```python
from build123d import *

# Parameters (mm, degrees)
BOSS_EXTRUDE1_DEPTH = 5
CUT_EXTRUDE1_DEPTH  = 5
CUT_EXTRUDE2_DEPTH  = 5
SKETCH7_R           = 1.5
CUT_EXTRUDE3_DEPTH  = 5
CUT_EXTRUDE4_DEPTH  = 5
SKETCH10_R          = 1.5
CUT_EXTRUDE5_DEPTH  = 5
CUT_EXTRUDE6_DEPTH  = 5
CUT_EXTRUDE7_DEPTH  = 5


with BuildPart() as part:
    # Sketch1 → Boss-Extrude1 (new body)
    with BuildSketch(Plane(origin=(0, 0, 0), x_dir=(1, 0, 0), z_dir=(0, 1, 0))):
        with BuildLine():
            Line((-4.859778007, 4.413916891), (128.140221993, 4.413916891))
            ThreePointArc((128.140221993, 4.413916891), (128.847328775, 4.121023672), (129.140221993, 3.413916891))
            Line((129.140221993, 3.413916891), (129.140221993, -144.586083109))
            ThreePointArc((129.140221993, -144.586083109), (128.847328775, -145.29318989), (128.140221993, -145.586083109))
            Line((128.140221993, -145.586083109), (-4.859778007, -145.586083109))
            ThreePointArc((-4.859778007, -145.586083109), (-5.566884788, -145.29318989), (-5.859778007, -144.586083109))
            Line((-5.859778007, -144.586083109), (-5.859778007, 3.413916891))
            ThreePointArc((-5.859778007, 3.413916891), (-5.566884788, 4.121023672), (-4.859778007, 4.413916891))
        make_face()
    extrude(amount=BOSS_EXTRUDE1_DEPTH)

    # Sketch3 → Cut-Extrude1 (cut)
    with BuildSketch(Plane(origin=(75.20450804, 5, 34.196611672), x_dir=(1, 0, 0), z_dir=(0, 1, 0))):
        with BuildLine():
            Line((45.935713953, -83.389471436), (45.935713953, -41.389471436))
            ThreePointArc((45.935713953, -41.389471436), (47.435713953, -39.889471436), (48.935713953, -41.389471436))
            Line((48.935713953, -41.389471436), (48.935713953, -83.389471436))
            ThreePointArc((48.935713953, -83.389471436), (47.435713953, -84.889471436), (45.935713953, -83.389471436))
        make_face()
        with BuildLine():
            Line((45.935713953, -31.389471436), (45.935713953, 10.610528564))
            ThreePointArc((45.935713953, 10.610528564), (47.435713953, 12.110528564), (48.935713953, 10.610528564))
            Line((48.935713953, 10.610528564), (48.935713953, -31.389471436))
            ThreePointArc((48.935713953, -31.389471436), (47.435713953, -32.889471436), (45.935713953, -31.389471436))
        make_face()
        with BuildLine():
            Line((-73.064286047, -84.889471436), (-73.064286047, -42.889471436))
            ThreePointArc((-73.064286047, -42.889471436), (-74.564286047, -41.389471436), (-76.064286047, -42.889471436))
            Line((-76.064286047, -42.889471436), (-76.064286047, -84.889471436))
            ThreePointArc((-76.064286047, -84.889471436), (-74.564286047, -86.389471436), (-73.064286047, -84.889471436))
        make_face()
        with BuildLine():
            Line((-73.064286047, -32.889471436), (-73.064286047, 9.110528564))
            ThreePointArc((-73.064286047, 9.110528564), (-74.564286047, 10.610528564), (-76.064286047, 9.110528564))
            Line((-76.064286047, 9.110528564), (-76.064286047, -32.889471436))
            ThreePointArc((-76.064286047, -32.889471436), (-74.564286047, -34.389471436), (-73.064286047, -32.889471436))
        make_face()
    extrude(amount=-CUT_EXTRUDE1_DEPTH, mode=Mode.SUBTRACT)

    # Sketch5 → Cut-Extrude2 (cut)
    with BuildSketch(Plane(origin=(75.20450804, 5, 34.196611672), x_dir=(1, 0, 0), z_dir=(0, 1, 0))):
        with BuildLine():
            Line((-60.064286047, -99.389471436), (-18.064286047, -99.389471436))
            ThreePointArc((-18.064286047, -99.389471436), (-16.564286047, -100.889471436), (-18.064286047, -102.389471436))
            Line((-18.064286047, -102.389471436), (-60.064286047, -102.389471436))
            ThreePointArc((-60.064286047, -102.389471436), (-61.564286047, -100.889471436), (-60.064286047, -99.389471436))
        make_face()
        with BuildLine():
            Line((-9.064286047, -99.389471436), (32.935713953, -99.389471436))
            ThreePointArc((32.935713953, -99.389471436), (34.435713953, -100.889471436), (32.935713953, -102.389471436))
            Line((32.935713953, -102.389471436), (-9.064286047, -102.389471436))
            ThreePointArc((-9.064286047, -102.389471436), (-10.564286047, -100.889471436), (-9.064286047, -99.389471436))
        make_face()
    extrude(amount=-CUT_EXTRUDE2_DEPTH, mode=Mode.SUBTRACT)

    # Sketch7 → Cut-Extrude3 (cut)
    with BuildSketch(Plane(origin=(75.20450804, 5, 34.196611672), x_dir=(1, 0, 0), z_dir=(0, 1, 0))):
        with Locations(Location((44.935713953, -98.389471436, 0), (0, 0, 270))):
            Circle(SKETCH7_R)
        with Locations(Location((44.935713953, 25.610528564, 0), (0, 0, 90))):
            Circle(SKETCH7_R)
        with Locations(Location((-74.064286047, 25.610528564, 0), (0, 0, 270))):
            Circle(SKETCH7_R)
        with BuildLine():
            Line((-72.564286047, -96.712473991), (-72.564286047, -100.066468882))
            ThreePointArc((-72.564286047, -100.066468882), (-74.064286047, -101.566468882), (-75.564286047, -100.066468882))
            Line((-75.564286047, -100.066468882), (-75.564286047, -96.712473991))
            ThreePointArc((-75.564286047, -96.712473991), (-74.064286047, -95.212473991), (-72.564286047, -96.712473991))
        make_face()
    extrude(amount=-CUT_EXTRUDE3_DEPTH, mode=Mode.SUBTRACT)

    # Sketch9 → Cut-Extrude4 (cut)
    with BuildSketch(Plane(origin=(75.20450804, 5, 34.196611672), x_dir=(1, 0, 0), z_dir=(0, 1, 0))):
        with BuildLine():
            Line((-40.064286047, -36.389471436), (12.935713953, -36.389471436))
            ThreePointArc((12.935713953, -36.389471436), (13.642820734, -36.682364655), (13.935713953, -37.389471436))
            Line((13.935713953, -37.389471436), (13.935713953, -55.389471436))
            ThreePointArc((13.935713953, -55.389471436), (13.642820734, -56.096578218), (12.935713953, -56.389471436))
            Line((12.935713953, -56.389471436), (-40.064286047, -56.389471436))
            ThreePointArc((-40.064286047, -56.389471436), (-40.771392828, -56.096578218), (-41.064286047, -55.389471436))
            Line((-41.064286047, -55.389471436), (-41.064286047, -37.389471436))
            ThreePointArc((-41.064286047, -37.389471436), (-40.771392828, -36.682364655), (-40.064286047, -36.389471436))
        make_face()
    extrude(amount=-CUT_EXTRUDE4_DEPTH, mode=Mode.SUBTRACT)

    # Sketch10 → Cut-Extrude5 (cut)
    with BuildSketch(Plane(origin=(0, 5, 0), x_dir=(1, 0, 0), z_dir=(0, 1, 0))):
        with Locations(Location((36.640221993, -5.586083109, 0), (0, 0, 270))):
            Circle(SKETCH10_R)
        with Locations(Location((86.640221993, -5.586083109, 0), (0, 0, 270))):
            Circle(SKETCH10_R)
        with Locations(Location((86.640221993, -55.586083109, 0), (0, 0, 270))):
            Circle(SKETCH10_R)
        with Locations(Location((36.640221993, -55.586083109, 0), (0, 0, 270))):
            Circle(SKETCH10_R)
    extrude(amount=-CUT_EXTRUDE5_DEPTH, mode=Mode.SUBTRACT)

    # Sketch11 → Cut-Extrude6 (cut)
    with BuildSketch(Plane(origin=(0, 5, 0), x_dir=(1, 0, 0), z_dir=(0, 1, 0))):
        with BuildLine():
            Line((32.140221993, -25.086083109), (32.140221993, -119.086083109))
            ThreePointArc((32.140221993, -119.086083109), (30.640221993, -120.586083109), (29.140221993, -119.086083109))
            Line((29.140221993, -119.086083109), (29.140221993, -25.086083109))
            ThreePointArc((29.140221993, -25.086083109), (30.640221993, -23.586083109), (32.140221993, -25.086083109))
        make_face()
        with BuildLine():
            Line((91.140221993, -25.086083109), (91.140221993, -119.086083109))
            ThreePointArc((91.140221993, -119.086083109), (92.640221993, -120.586083109), (94.140221993, -119.086083109))
            Line((94.140221993, -119.086083109), (94.140221993, -25.086083109))
            ThreePointArc((94.140221993, -25.086083109), (92.640221993, -23.586083109), (91.140221993, -25.086083109))
        make_face()
    extrude(amount=-CUT_EXTRUDE6_DEPTH, mode=Mode.SUBTRACT)

    # Sketch12 → Cut-Extrude7 (cut)
    with BuildSketch(Plane(origin=(0, 5, 0), x_dir=(1, 0, 0), z_dir=(0, 1, 0))):
        with BuildLine():
            Line((22.394580423, -97.440920872), (8.394580423, -97.440920872))
            ThreePointArc((8.394580423, -97.440920872), (7.687473642, -97.148027653), (7.394580423, -96.440920872))
            Line((7.394580423, -96.440920872), (7.394580423, -88.440920872))
            ThreePointArc((7.394580423, -88.440920872), (7.687473642, -87.733814091), (8.394580423, -87.440920872))
            Line((8.394580423, -87.440920872), (22.394580423, -87.440920872))
            ThreePointArc((22.394580423, -87.440920872), (23.101687204, -87.733814091), (23.394580423, -88.440920872))
            Line((23.394580423, -88.440920872), (23.394580423, -96.440920872))
            ThreePointArc((23.394580423, -96.440920872), (23.101687204, -97.148027653), (22.394580423, -97.440920872))
        make_face()
        with BuildLine():
            Line((100.885863564, -87.440920872), (114.885863564, -87.440920872))
            ThreePointArc((114.885863564, -87.440920872), (115.592970345, -87.733814091), (115.885863564, -88.440920872))
            Line((115.885863564, -88.440920872), (115.885863564, -96.440920872))
            ThreePointArc((115.885863564, -96.440920872), (115.592970345, -97.148027653), (114.885863564, -97.440920872))
            Line((114.885863564, -97.440920872), (100.885863564, -97.440920872))
            ThreePointArc((100.885863564, -97.440920872), (100.178756783, -97.148027653), (99.885863564, -96.440920872))
            Line((99.885863564, -96.440920872), (99.885863564, -88.440920872))
            ThreePointArc((99.885863564, -88.440920872), (100.178756783, -87.733814091), (100.885863564, -87.440920872))
        make_face()
    extrude(amount=-CUT_EXTRUDE7_DEPTH, mode=Mode.SUBTRACT)


solid = part.part
```
The listing builds one solid part. Answer for the finished solid, in the listing's coordinates (mm). A direction names the side the tool comes from. Give positions to 0.01 mm unless a question says otherwise; leave off trailing zeros. Loops run counter-clockwise (first coordinate to the right, second up) from the corner with the lowest first, then second, coordinate; pieces in that order, holes last. Notation, with made-up numbers: (61.5, 17) - (101.5, 17) arc R23 ccw to (101.5, 45) - close; hole circle Ø4 at (-23.75, -27.5). An arc over 180 degrees is marked (long way). Return JSON: item names as keys, results as strings. Group by question number.
1. Find section B-B (x = 69). Write down the section's boundary in (y, z), then the cut area to 3 significant figures.
2. Straight lines are drawn through the part: line 1 (X direction, y = 4.7, z = 63.5); line 2 (Z direction, x = 108, y = 1.9); line 3 (X direction, y = 2.2, z = 81). For each, find the intervals that lie inside material, in ascending order. Write a range as [from, to].
3. Find section D-D (y = 2.6). State how many separate pieces and enclosed holes the cut face has, then the cut area to 3 significant figures.
4. Determine the mould class of faces 3 (the flat face through (62, 3, 90.586)), 4 (the flat face through (124.14, 3, 44)), 5 (the flat face through (63, 2, 145.586)) for opening direction X: pulls with the +X half, pulls with the -X half, needs draft (parallel to the pull), parting line crosses it, or undercut.
5. Find section C-C (x = 105.5). Write down the section's boundary in (y, z), then the cut area to 3 significant figures.
6. Given pin 1 Ø2 at (x, z) = (42, 13.5) entering from -Y, flat-ended and moving along its own axis, determine where the tip first touches the part or whether it passes through.
7. Find section A-A (z = 29). Write down the section's boundary in (x, y), then the cut area to 3 significant figures.
8. Which of the six approach directions +Z, -Z, +X, -X, +Y, -Y give full straight-line access (tool end or side, diameter ignored) to faces 1 (the flat face through (124.14, 3, 96)), 2 (the flat face through (63, 0, 70))?
Verdict:
{
 "1": {"outline": "(0, -4.41) - (5, -4.41) - (5, 70.59) - (0, 70.59) - close; (0, 90.59) - (5, 90.59) - (5, 133.59) - (0, 133.59) - close; (0, 136.59) - (5, 136.59) - (5, 145.59) - (0, 145.59) - close", "area": "635 mm^2"},
 "2": {"line 1": "x = [-5.86, -0.86], [2.14, 29.14], [32.14, 91.14], [94.14, 121.14], [124.14, 129.14]", "line 2": "z = [-4.41, 87.44], [97.44, 133.59], [136.59, 145.59]", "line 3": "x = [-5.86, -0.86], [2.14, 29.14], [32.14, 34.14], [89.14, 91.14], [94.14, 121.14], [124.14, 129.14]"},
 "3": {"separate pieces": "1", "enclosed holes": "19", "area": "17,400 mm^2"},
 "4": {"face 3": "undercut", "face 4": "undercut", "face 5": "needs draft"},
 "5": {"outline": "(0, -4.41) - (5, -4.41) - (5, 87.44) - (0, 87.44) - close; (0, 97.44) - (5, 97.44) - (5, 133.59) - (0, 133.59) - close; (0, 136.59) - (5, 136.59) - (5, 145.59) - (0, 145.59) - close", "area": "685 mm^2"},
 "6": {"pin 1": "stops at y = 0"},
 "7": {"outline": "(-5.86, 0) - (-0.86, 0) - (-0.86, 5) - (-5.86, 5) - close; (2.14, 0) - (29.14, 0) - (29.14, 5) - (2.14, 5) - close; (32.14, 0) - (91.14, 0) - (91.14, 5) - (32.14, 5) - close; (94.14, 0) - (121.14, 0) - (121.14, 5) - (94.14, 5) - close; (124.14, 0) - (129.14, 0) - (129.14, 5) - (124.14, 5) - close", "area": "615 mm^2"},
 "8": {"face 1": "+Y, -Y", "face 2": "+Z, -Z, +X, -X, -Y"}
}
